from build123d import *

# Parameters (mm, degrees)
SKETCH1_R = 0.8001


with BuildPart() as part:
    # Sweep1: sweep along a path in Sketch2
    with BuildLine(Plane(origin=(0, 0, 0), x_dir=(0, 0, -1), z_dir=(1, 0, 0))) as sweep1_path:
        Line((0, 0), (30.1498, 0))
        ThreePointArc((30.1498, 0), (34.009420782, 4.926282123), (28.302700663, 7.494992619))
        Line((28.302700663, 7.494992619), (18.916315959, 2.569392085))
        ThreePointArc((18.916315959, 2.569392085), (17.948121595, 2.404428196), (17.068166617, 2.840653653))
        ThreePointArc((17.068166617, 2.840653653), (14.2875, 3.9751), (11.506833383, 2.840653653))
        ThreePointArc((11.506833383, 2.840653653), (10.595153346, 2.400098126), (9.60259352, 2.600284671))
        Line((9.60259352, 2.600284671), (1.74625, 7.136146718))
    # Sketch1 → Sweep1 (sweep)
    with BuildSketch(Plane.XY):
        Circle(SKETCH1_R)
    sweep(path=sweep1_path.line)


solid = part.part
Check sheet for the modelled part. Datum: model origin and axes. Units: mm. Give positions to 0.01 mm unless a question says otherwise; leave off trailing zeros. Loops run counter-clockwise (first coordinate to the right, second up) from the corner with the lowest first, then second, coordinate; pieces in that order, holes last. Notation, with made-up numbers: M 25,-14.5 L 63,-14.5 A10 ccw 63,4.5 Z; hole C 66,-9 d10. An arc over 180 degrees is marked long. Return JSON: item names as keys, results as strings. Group by question number.
1. Thickness scan on L1, parallel to Z at x = -0.3, y = 4; L2, parallel to Z at x = 0.05, y = 5.25; L3, parallel to Z at x = 0.2, y = 2. Record the ranges inside material, lowest first.
2. Cross-section at A-A on x = 0.4. Record the boundary of the cut face in (y, z).
3. Mould release check, pull along Z, two halves, no side actions. Record for faces 1 (the flat face through (0, 0, 0)), 2 (the cylindrical face through (-0.63, 0.49, -15.29)), 3 (the cylindrical face through (-0.17, 4.22, -5.23)): released by +Z, released by -Z, zero draft, split by the parting line, or undercut.
Return value:
{
 "1": {"L1": "-34.87 to -33.38, -23.24 to -20.05, -16.79 to -11.79, -8.66 to -5.69", "L2": "-34.75 to -33.06, -25.74 to -22.31, -6.61 to -3.42", "L3": "-34.47 to -32.67, -19.5 to -16.88, -11.69 to -9.09"},
 "2": {"outline": "M -0.69,-30.15 A4.67 ccw long 8.11,-27.98 L 3.18,-18.59 A0.89 cw 3.34,-17.55 A4.67 ccw 3.34,-11.02 A0.89 cw 3.2,-9.95 L 7.74,-2.09 L 6.54,-1.4 L 2,-9.26 A2.28 ccw 2.35,-11.99 A3.28 cw 2.35,-16.58 A2.28 ccw 1.96,-19.24 L 6.88,-28.62 A3.28 cw long 0.69,-30.15 L 0.69,0 L -0.69,0 Z"},
 "3": {"face 1": "released by +Z", "face 2": "zero draft", "face 3": "undercut"}
}
